Part print with two shaded views. Sizes in mm from the minimum x, y, z corner. A direction names the side the tool comes from. Give positions to 0.01 mm unless a question says otherwise; leave off trailing zeros. Write each loop counter-clockwise with the first axis right and the second up, starting at its lowest first coordinate (ties: lowest second). Pieces come first, ordered by that corner, then holes. Notation, with made-up numbers: (45, -13) - (81, -13) arc R17 ccw to (81, 11) - close; hole circle Ø11 at (12, 31.25). An arc over 180 degrees is marked (long way). Answer as a JSON object with one key per item and string values.
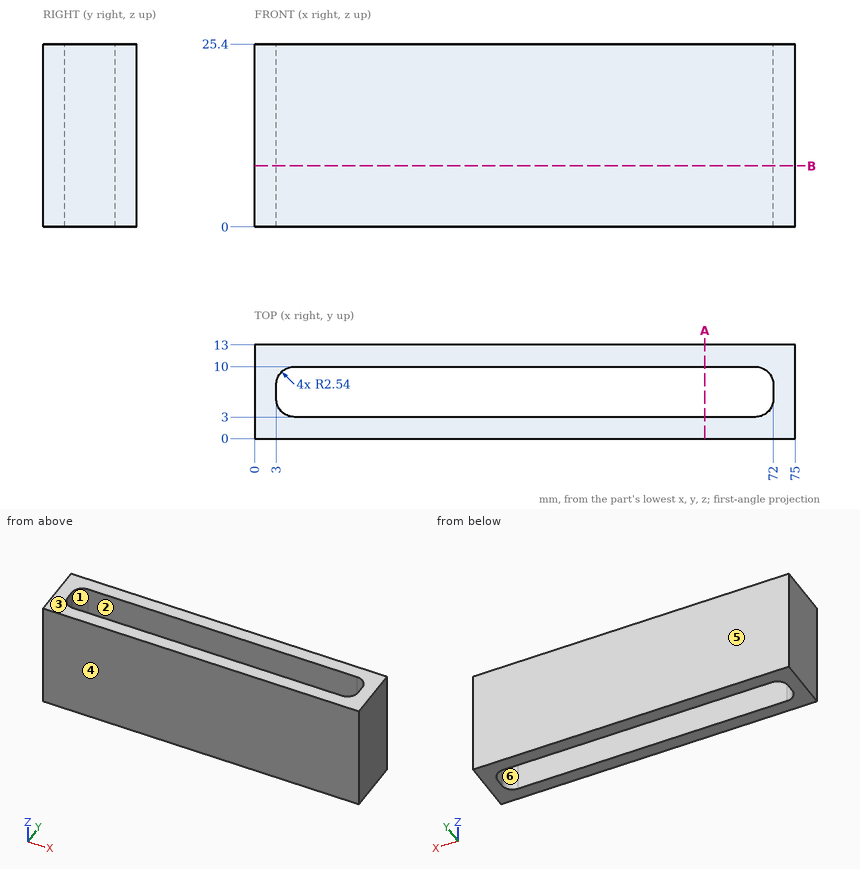
(1) Saw through at B-B, the plane z = 8.5. Give the cut face in (x, y).
Answer key:
{"outline": "(0, 0) - (75, 0) - (75, 13) - (0, 13) - close; hole (3, 5.54) arc R2.54 ccw to (5.54, 3) - (69.46, 3) arc R2.54 ccw to (72, 5.54) - (72, 7.46) arc R2.54 ccw to (69.46, 10) - (5.54, 10) arc R2.54 ccw to (3, 7.46) - close"}
(2) 3-axis set-ups, long thin cutter, end or side, ignore diameter. For the marked faces 5 and 6: which of +Z, -Z, +X, -X, +Y, -Y reach the whole face in a straight line?
Answer key:
{"face 5": "+Z, -Z, +X, -X, +Y", "face 6": "+Z, -Z"}
(3) Pull direction Y, two halves, no side cores. Call the marked faces 1, 2, 3 and 4: pulls with the +Y half, pulls with the -Y half, needs draft (parallel to the pull), parting line crosses it, or undercut.
Answer key:
{"face 1": "undercut", "face 2": "undercut", "face 3": "needs draft", "face 4": "pulls with the -Y half"}
(4) Saw through at A-A, the plane x = 62.5. Give the cut face in (y, z).
Answer key:
{"outline": "(0, 0) - (3, 0) - (3, 25.4) - (0, 25.4) - close; (10, 0) - (13, 0) - (13, 25.4) - (10, 25.4) - close"}
(5) Probe L1, parallel to X at y = 7.75, z = 5; L2, parallel to Y at x = 55, z = 11.5; L3, parallel to X at y = 4.25, z = 6.75. List the from-to ranges inside material, lowest first. Write a range as [from, to].
Answer key:
{"L1": "x = [0, 3.02], [71.98, 75]", "L2": "y = [0, 3], [10, 13]", "L3": "x = [0, 3.35], [71.65, 75]"}
